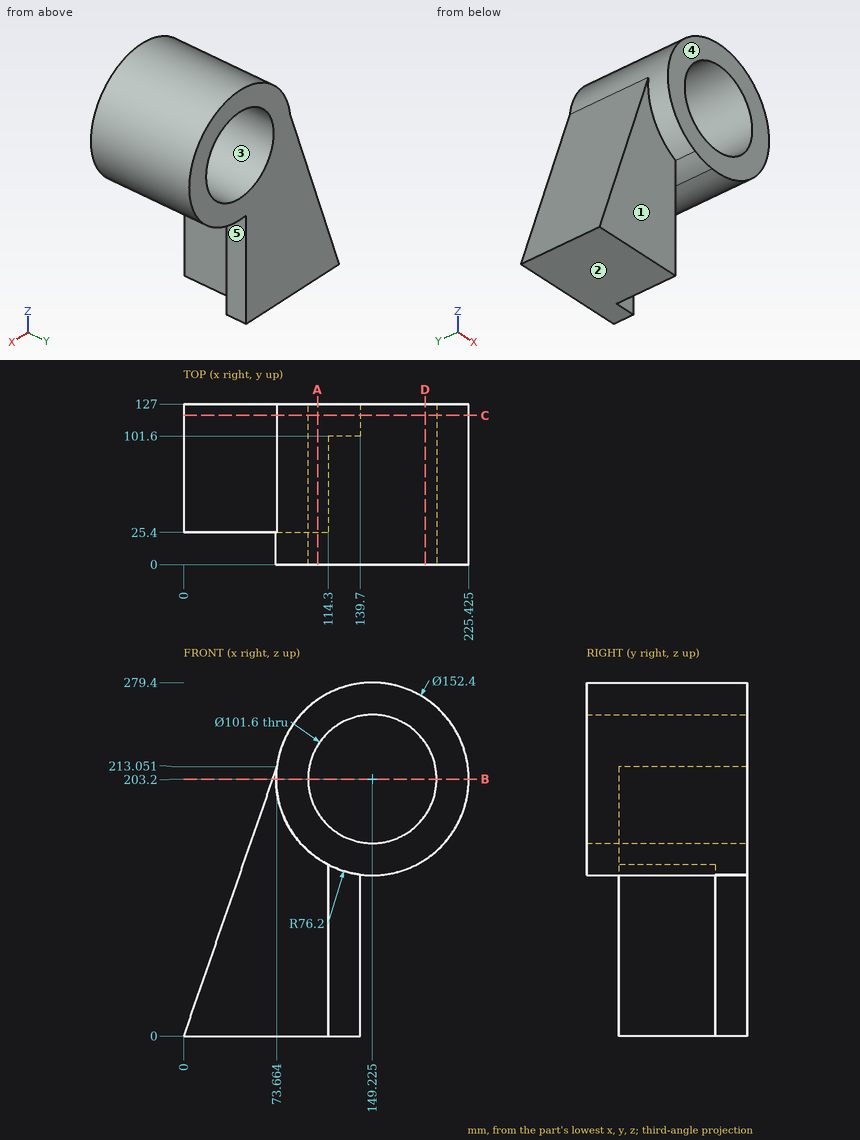
Verification items for this drawing (mm, ordinates from the low corner). A direction names the side the tool comes from. Round coordinates to 2 decimals unless told otherwise and drop trailing zeros. Loops run counter-clockwise (first coordinate to the right, second up) from the corner with the lowest first, then second, coordinate; pieces in that order, holes last. Notation, with made-up numbers: (81.5, -25.75) - (138.5, -25.75) arc R11 ccw to (138.5, -8.75) - close; hole circle Ø6 at (-11, -37). An arc over 180 degrees is marked (long way). Answer as CSV lines item,"result". Start each with the question number.
Item 1: Depth check by flat-ended pin: P1, Ø12.5, axis at y = 120, z = 42, coming from the +X side; P2, Ø20.5, axis at x = 130, z = 76, coming from the -Y side; P3, Ø8, axis at x = 154.5, y = 88, coming from the -Z side. Enter the tip coordinate at first touch or a pass-through.
Item 2: Section check C-C (y = 118). Record the boundary of the cut face in (x, z) (1 decimal).
Item 3: Scan lines: line 1 (Z direction, x = 151, y = 41.5); line 2 (Z direction, x = 118, y = 103.5); line 3 (Y direction, x = 20, z = 50.5). Record each from-to range of solid material in increasing order. Write a range as [from, to].
Item 4: Section check B-B (z = 203.2). Record the boundary of the cut face in (x, y) (1 decimal).
Item 5: Section check D-D (x = 191). Record the boundary of the cut face in (y, z) (1 decimal).
Item 6: Section check A-A (x = 106). Record the boundary of the cut face in (y, z), and give its area (3 significant figures).
Item 7: Release check for a two-part mould opening along X. For the marked faces 3, 4 and 5 record: +X half, -X half, draft (parallel to the pull), parting line (faces both ways), or undercut.
Item 8: Set-up check for the marked faces 1 and 2: record each of +Z, -Z, +X, -X, +Y, -Y from which the full face is reachable in a straight line by a thin tool's end or side.
Report:
1,P1,"stops at x = 139.7"
1,P2,"stops at y = 101.6"
1,P3,"stops at z = 127.01"
2,outline,"(0, 0) - (139.7, 0) - (139.7, 127.6) arc R76.2 ccw (long way) to (73.7, 213.1) - close; hole circle Ø101.6 at (149.2, 203.2)"
3,line 1,"z = [127.02, 152.43], [253.97, 279.38]"
3,line 2,"z = [0, 163.13], [243.27, 272.71]"
3,line 3,"y = [25.4, 127]"
4,outline,"(70.3, 25.4) - (73, 25.4) - (73, 0) - (98.4, 0) - (98.4, 127) - (70.3, 127) - close; (200, 0) - (225.4, 0) - (225.4, 127) - (200, 127) - close"
5,outline,"(0, 139.5) - (127, 139.5) - (127, 174.3) - (0, 174.3) - close; (0, 232.1) - (127, 232.1) - (127, 266.9) - (0, 266.9) - close"
6,outline,"(0, 140.45) - (25.4, 140.45) - (25.4, 0) - (127, 0) - (127, 176.51) - (0, 176.51) - close; (0, 229.89) - (127, 229.89) - (127, 265.95) - (0, 265.95) - close"
6,area,"23,400 mm2"
7,face 3,"undercut"
7,face 4,"draft"
7,face 5,"+X half"
8,face 1,"-Z, -X, -Y"
8,face 2,"-Z, +X, -X, +Y, -Y"
